```python
from build123d import *

# Parameters (mm, degrees)
MODEL_W                 = 3
MODEL_H                 = 3
SALIENTE_EXTRUIR1_DEPTH = 3


with BuildPart() as part:
    # Model → Saliente-Extruir1 (new body)
    with BuildSketch(Plane.XY):
        with BuildLine():
            Line((12.603795093, 298.783404974), (21.603795093, 298.783404974))
            ThreePointArc((21.603795093, 298.783404974), (26.103795093, 294.283404974), (21.603795093, 289.783404974))
            Line((21.603795093, 289.783404974), (12.603795093, 289.783404974))
            ThreePointArc((12.603795093, 289.783404974), (8.103795093, 294.283404974), (12.603795093, 298.783404974))
        make_face()
        with Locations((12.603795093, 294.283404974)):
            Rectangle(MODEL_W, MODEL_H, mode=Mode.SUBTRACT)
        with Locations((21.603795093, 294.283404974)):
            Rectangle(MODEL_W, MODEL_H, mode=Mode.SUBTRACT)
    extrude(amount=SALIENTE_EXTRUIR1_DEPTH)


solid = part.part
```
The model under review builds one solid part; all positions refer to its coordinate system, in mm. A direction names the side the tool comes from. Round coordinates to 2 decimals unless told otherwise and drop trailing zeros. Loops run counter-clockwise (first coordinate to the right, second up) from the corner with the lowest first, then second, coordinate; pieces in that order, holes last.
1) Tool access review of faces 1 (the face through (22, 292.783, 1)), 2 (the face through (26.103, 294.382, 1.479)): name each direction out of +Z, -Z, +X, -X, +Y, -Y from which nothing blocks a thin tool from reaching the whole face with its end or side.
Values follow:
face 1: +Z, -Z
face 2: +Z, -Z, +X
2) Clearance check with a flat-ended pin moving along its axis: P1, Ø1.5, axis at y = 294.5, z = 1.5, coming from the -X side. State where the tip first meets the part, or that it passes through.
Values follow:
P1: stops at x = 8.1
3) Consider section C-C on x = 24.25. State the section outline as (y, z) points.
Values follow:
outline: (290.64, 0) - (297.92, 0) - (297.92, 3) - (290.64, 3) - close
4) Consider section A-A on z = 0.9. State the section outline as (x, y) points.
Values follow:
outline: (12.6, 289.78) - (21.6, 289.78) arc R4.5 ccw to (21.6, 298.78) - (12.6, 298.78) arc R4.5 ccw to start; hole (11.1, 292.78) - (14.1, 292.78) - (14.1, 295.78) - (11.1, 295.78) - close; hole (20.1, 292.78) - (23.1, 292.78) - (23.1, 295.78) - (20.1, 295.78) - close
5) Wall thickness on line 1 along Y through (x, z) = (20.5, 0.45); line 2 along X through (y, z) = (295.25, 0.3); line 3 along X through (y, z) = (293.75, 0.1): over which ranges is each line inside the solid? List them lowest first.
Values follow:
line 1: y = 289.78 to 292.78, 295.78 to 298.78
line 2: x = 8.21 to 11.1, 14.1 to 20.1, 23.1 to 26
line 3: x = 8.14 to 11.1, 14.1 to 20.1, 23.1 to 26.07
6) The part is to be moulded in two halves that separate along X. For faces 3 (the face through (11.104, 294, 1)), 4 (the face through (17, 289.783, 1)), 5 (the face through (8.105, 294.184, 1.479)), say which applies: pulls with the +X half, pulls with the -X half, needs draft (parallel to the pull), parting line crosses it, or undercut.
Values follow:
face 3: undercut
face 4: needs draft
face 5: pulls with the -X half
7) Consider section B-B on y = 293.5. State the section outline as (x, z) points, then the cut area to 3 significant figures.
Values follow:
outline: (8.17, 0) - (11.1, 0) - (11.1, 3) - (8.17, 3) - close; (14.1, 0) - (20.1, 0) - (20.1, 3) - (14.1, 3) - close; (23.1, 0) - (26.04, 0) - (26.04, 3) - (23.1, 3) - close
area: 35.6 mm2
8) Consider section D-D on y = 298.25. State the section outline as (x, z) points.
Values follow:
outline: (10.48, 0) - (23.73, 0) - (23.73, 3) - (10.48, 3) - close
